Verification items for the finished model (mm, model axes). A direction names the side the tool comes from. Give positions to 0.01 mm unless a question says otherwise; leave off trailing zeros. Order: outer loops, then holes, each group sorted by start corner. A loop starts at its lowest first (then second) coordinate and runs counter-clockwise, first axis right, second up. Notation, with made-up numbers: (31, -29.75) -> (63, -29.75) arc R13 cw to (63, -24.75) -> close; hole circle Ø8 at (72, 3). An arc over 180 degrees is marked (long way). One line per question, with ' | ' between items. Start each with the question number.
Q1. Section check B-B on x = -33. Record the cut outline in (y, z), plus the area to 3 significant figures.
Q2. Section check D-D on z = -13. Record the cut outline in (x, y).
Q3. Go/stop test with flat-tipped pins: pin 1 (0.6 mm diameter, centred on y = -26, z = -15, fed in from +X); pin 2 (4 mm diameter, centred on x = -44.5, y = -23, fed in from +Z); pin 3 (0.9 mm diameter, centred on y = -26.5, z = -17, fed in from -X). Record where each tip stops, or that it passes through.
Q4. Material ranges on probe 1 along X at (y, z) = (-9, -14.5); probe 2 along Y at (x, z) = (-40, -10.25); probe 3 along Y at (x, z) = (9, -19.5), recorded low to high. Write a range as [from, to].
Q5. Section check C-C on z = -7.75. Record the cut outline in (x, y), plus the area to 3 significant figures.
Q6. Section check A-A on y = 3.5. Record the cut outline in (x, z), plus the area to 3 significant figures.
Q7. Mould release check, pull along Y, two halves, no side actions. Record for faces 1 (the flat face through (-44, -21, -11.25)), 2 (the flat face through (-49, 1, -2)), 3 (the flat face through (-44, 22.7, -11.25)), 4 (the flat face through (-10, 28.924, -11)): released by +Y, released by -Y, zero draft, split by the parting line, or undercut.
Q8. Access from +Z, -Z, +X, -X, +Y, -Y to the whole of each face (thin tool, end or side, straight path). Record for faces 5 (the flat face through (-10, -25.976, -20)), 6 (the flat face through (29.665, 0, -3)), 7 (the cylindrical face through (-43.843, 24.1, -15.071)), 8 (the flat face through (31.165, 0, -11)), 9 (the flat face through (-7, -26, -18.312)).
from build123d import *

# Parameters (mm, degrees)
BOSS_EXTRUDE1_START = -2
SKETCH1_W           = 81.4
SKETCH1_H           = 56.4
SKETCH1_W_2         = 75.4
SKETCH1_H_2         = 50.4
BOSS_EXTRUDE1_DEPTH = 27
FILLET1_R           = 3
SKETCH2_R           = 1.3
CUT_EXTRUDE1_DEPTH  = 2
CUT_EXTRUDE2_START  = -17
SKETCH2_3_R         = 1.3
CUT_EXTRUDE2_DEPTH  = 10
BOSS_EXTRUDE2_START = -7.25
SKETCH3_R           = 1.25
BOSS_EXTRUDE2_DEPTH = 7.75
CUT_EXTRUDE3_DEPTH  = 28.2
CUT_EXTRUDE4_START  = -8
CUT_EXTRUDE4_DEPTH  = 8


with BuildPart() as part:
    # Sketch1 → Boss-Extrude1 (new body)
    with BuildSketch(Plane.XY.offset(BOSS_EXTRUDE1_START)):
        with Locations((-9.535141298, 0.724362859)):
            Rectangle(SKETCH1_W, SKETCH1_H)
        with Locations((-9.535141298, 0.724362859)):
            Rectangle(SKETCH1_W_2, SKETCH1_H_2, mode=Mode.SUBTRACT)
    extrude(amount=-BOSS_EXTRUDE1_DEPTH)

    # Fillet1
    fillet1_edges = [part.edges().sort_by_distance(p)[0] for p in [
        (-50.235141298, -27.475637141, -15.5),
        (-50.235141298, 28.924362859, -15.5),
        (31.164858702, 28.924362859, -15.5),
        (31.164858702, -27.475637141, -15.5),
    ]]
    fillet(fillet1_edges, radius=FILLET1_R)

    # Sketch2 → Cut-Extrude1 (cut)
    with BuildSketch(Plane.XY.offset(-2)):
        with Locations((25.964858702, -22.275637141)):
            Circle(SKETCH2_R)
        with BuildLine():
            Line((28.164858702, 27.424362859), (-47.235141298, 27.424362859))
            ThreePointArc((-47.235141298, 27.424362859), (-48.29580147, 26.985023031), (-48.735141298, 25.924362859))
            Line((-48.735141298, 25.924362859), (-48.735141298, -24.475637141))
            ThreePointArc((-48.735141298, -24.475637141), (-48.29580147, -25.536297313), (-47.235141298, -25.975637141))
            Line((-47.235141298, -25.975637141), (28.164858702, -25.975637141))
            ThreePointArc((28.164858702, -25.975637141), (29.225518873, -25.536297313), (29.664858702, -24.475637141))
            Line((29.664858702, -24.475637141), (29.664858702, 25.924362859))
            ThreePointArc((29.664858702, 25.924362859), (29.225518873, 26.985023031), (28.164858702, 27.424362859))
        make_face()
    extrude(amount=-CUT_EXTRUDE1_DEPTH, mode=Mode.SUBTRACT)

    # Sketch2<3> → Cut-Extrude2 (cut)
    with BuildSketch(Plane.XY.offset(-2).offset(CUT_EXTRUDE2_START)):
        with BuildLine():
            Line((28.164858702, 27.424362859), (-47.235141298, 27.424362859))
            ThreePointArc((-47.235141298, 27.424362859), (-48.29580147, 26.985023031), (-48.735141298, 25.924362859))
            Line((-48.735141298, 25.924362859), (-48.735141298, -24.475637141))
            ThreePointArc((-48.735141298, -24.475637141), (-48.29580147, -25.536297313), (-47.235141298, -25.975637141))
            Line((-47.235141298, -25.975637141), (28.164858702, -25.975637141))
            ThreePointArc((28.164858702, -25.975637141), (29.225518873, -25.536297313), (29.664858702, -24.475637141))
            Line((29.664858702, -24.475637141), (29.664858702, 25.924362859))
            ThreePointArc((29.664858702, 25.924362859), (29.225518873, 26.985023031), (28.164858702, 27.424362859))
        make_face()
        with Locations((25.964858702, 23.724362859)):
            Circle(SKETCH2_3_R, mode=Mode.SUBTRACT)
        with Locations((-45.035141298, 23.724362859)):
            Circle(SKETCH2_3_R, mode=Mode.SUBTRACT)
        with Locations((-45.035141298, -22.275637141)):
            Circle(SKETCH2_3_R, mode=Mode.SUBTRACT)
        with Locations((25.964858702, -22.275637141)):
            Circle(SKETCH2_3_R, mode=Mode.SUBTRACT)
    extrude(amount=-CUT_EXTRUDE2_DEPTH, mode=Mode.SUBTRACT)

    # Sketch3 → Boss-Extrude2 (add)
    # profile 1 of 4: a face of its own
    with BuildSketch(Plane.XY.offset(-4).offset(BOSS_EXTRUDE2_START)):
        with BuildLine():
            Line((-47.235141298, -24.475637141), (-42.835141298, -24.475637141))
            ThreePointArc((-42.835141298, -24.475637141), (-42.160702776, -23.466268561), (-41.923871461, -22.275637141))
            ThreePointArc((-41.923871461, -22.275637141), (-43.844509878, -19.401198618), (-47.235141298, -20.075637141))
            Line((-47.235141298, -20.075637141), (-47.235141298, -24.475637141))
        make_face()
        with Locations((-45.035141298, -22.275637141)):
            Circle(SKETCH3_R, mode=Mode.SUBTRACT)
    # profile 2 of 4: a face of its own
    with BuildSketch(Plane.XY.offset(-4).offset(BOSS_EXTRUDE2_START)):
        with BuildLine():
            ThreePointArc((-41.923871461, 23.724362859), (-42.160702776, 24.914994279), (-42.835141298, 25.924362859))
            Line((-42.835141298, 25.924362859), (-47.235141298, 25.924362859))
            Line((-47.235141298, 25.924362859), (-47.235141298, 21.524362859))
            ThreePointArc((-47.235141298, 21.524362859), (-43.844509878, 20.849924336), (-41.923871461, 23.724362859))
        make_face()
        with Locations((-45.035141298, 23.724362859)):
            Circle(SKETCH3_R, mode=Mode.SUBTRACT)
    # profile 3 of 4: a face of its own
    with BuildSketch(Plane.XY.offset(-4).offset(BOSS_EXTRUDE2_START)):
        with BuildLine():
            ThreePointArc((23.764858702, 25.924362859), (23.764858702, 21.524362859), (28.164858702, 21.524362859))
            Line((28.164858702, 21.524362859), (28.164858702, 25.924362859))
            Line((28.164858702, 25.924362859), (23.764858702, 25.924362859))
        make_face()
        with Locations((25.964858702, 23.724362859)):
            Circle(SKETCH3_R, mode=Mode.SUBTRACT)
    # profile 4 of 4: a face of its own
    with BuildSketch(Plane.XY.offset(-4).offset(BOSS_EXTRUDE2_START)):
        with BuildLine():
            Line((23.764858702, -24.475637141), (28.164858702, -24.475637141))
            Line((28.164858702, -24.475637141), (28.164858702, -20.075637141))
            ThreePointArc((28.164858702, -20.075637141), (23.764858702, -20.075637141), (23.764858702, -24.475637141))
        make_face()
        with Locations((25.964858702, -22.275637141)):
            Circle(SKETCH3_R, mode=Mode.SUBTRACT)
    extrude(amount=-BOSS_EXTRUDE2_DEPTH)

    # Sketch5 → Cut-Extrude3 (cut)
    with BuildSketch(Plane.XZ.offset(27.475637141)):
        with BuildLine():
            Line((-10.285143265, -18.312481798), (-3.785143265, -18.312481798))
            ThreePointArc((-3.785143265, -18.312481798), (-3.184102501, -18.063522562), (-2.935143265, -17.462481798))
            Line((-2.935143265, -17.462481798), (-2.935143265, -16.642481798))
            ThreePointArc((-2.935143265, -16.642481798), (-3.025595699, -16.260922505), (-3.277702075, -15.960570192))
            Line((-3.277702075, -15.960570192), (-3.489691711, -15.80281914))
            ThreePointArc((-3.489691711, -15.80281914), (-3.534181071, -15.749815791), (-3.550143265, -15.682481798))
            Line((-3.550143265, -15.682481798), (-3.550143265, -14.962481798))
            ThreePointArc((-3.550143265, -14.962481798), (-3.799102501, -14.361441034), (-4.400143265, -14.112481798))
            Line((-4.400143265, -14.112481798), (-9.670143265, -14.112481798))
            ThreePointArc((-9.670143265, -14.112481798), (-10.271184029, -14.361441034), (-10.520143265, -14.962481798))
            Line((-10.520143265, -14.962481798), (-10.520143265, -15.682481798))
            ThreePointArc((-10.520143265, -15.682481798), (-10.53610546, -15.749815791), (-10.58059482, -15.80281914))
            Line((-10.58059482, -15.80281914), (-10.792584456, -15.960570192))
            ThreePointArc((-10.792584456, -15.960570192), (-11.044690832, -16.260922505), (-11.135143265, -16.642481798))
            Line((-11.135143265, -16.642481798), (-11.135143265, -17.462481798))
            ThreePointArc((-11.135143265, -17.462481798), (-10.886184029, -18.063522562), (-10.285143265, -18.312481798))
        make_face()
    extrude(amount=-CUT_EXTRUDE3_DEPTH, mode=Mode.SUBTRACT)

    # Sketch6 → Cut-Extrude4 (cut)
    with BuildSketch(Plane(origin=(0, 0, -29), x_dir=(-1, 0, 0), z_dir=(0, 0, -1)).offset(CUT_EXTRUDE4_START)):
        with BuildLine():
            Line((50.235141298, -24.475637141), (50.235141298, 25.924362859))
            ThreePointArc((50.235141298, 25.924362859), (49.356461642, 28.045683202), (47.235141298, 28.924362859))
            Line((47.235141298, 28.924362859), (-28.164858702, 28.924362859))
            ThreePointArc((-28.164858702, 28.924362859), (-30.286179045, 28.045683202), (-31.164858702, 25.924362859))
            Line((-31.164858702, 25.924362859), (-31.164858702, -24.475637141))
            ThreePointArc((-31.164858702, -24.475637141), (-30.286179045, -26.596957485), (-28.164858702, -27.475637141))
            Line((-28.164858702, -27.475637141), (47.235141298, -27.475637141))
            ThreePointArc((47.235141298, -27.475637141), (49.356461642, -26.596957485), (50.235141298, -24.475637141))
        make_face()
        with BuildLine():
            Line((-29.664858702, 25.924362859), (-29.664858702, -24.475637141))
            ThreePointArc((-29.664858702, -24.475637141), (-29.225518873, -25.536297313), (-28.164858702, -25.975637141))
            Line((-28.164858702, -25.975637141), (47.235141298, -25.975637141))
            ThreePointArc((47.235141298, -25.975637141), (48.29580147, -25.536297313), (48.735141298, -24.475637141))
            Line((48.735141298, -24.475637141), (48.735141298, 25.924362859))
            ThreePointArc((48.735141298, 25.924362859), (48.29580147, 26.985023031), (47.235141298, 27.424362859))
            Line((47.235141298, 27.424362859), (-28.164858702, 27.424362859))
            ThreePointArc((-28.164858702, 27.424362859), (-29.225518873, 26.985023031), (-29.664858702, 25.924362859))
        make_face(mode=Mode.SUBTRACT)
    extrude(amount=CUT_EXTRUDE4_DEPTH, mode=Mode.SUBTRACT)


solid = part.part
Filled in:
1) outline: (-27.48, -21) -> (-25.98, -21) -> (-25.98, -19) -> (-24.48, -19) -> (-24.48, -4) -> (-25.98, -4) -> (-25.98, -2) -> (-27.48, -2) -> close; (25.92, -19) -> (27.42, -19) -> (27.42, -21) -> (28.92, -21) -> (28.92, -2) -> (27.42, -2) -> (27.42, -4) -> (25.92, -4) -> close | area: 102 mm²
2) outline: (-50.24, -24.48) arc R3 ccw to (-47.24, -27.48) -> (28.16, -27.48) arc R3 ccw to (31.16, -24.48) -> (31.16, 25.92) arc R3 ccw to (28.16, 28.92) -> (-47.24, 28.92) arc R3 ccw to (-50.24, 25.92) -> close; hole (-47.24, -20.08) arc R3.11 cw to (-42.84, -24.48) -> (23.76, -24.48) arc R3.11 cw to (28.16, -20.08) -> (28.16, 21.52) arc R3.11 cw to (23.76, 25.92) -> (-42.84, 25.92) arc R3.11 cw to (-47.24, 21.52) -> close; hole circle Ø2.5 at (-45.04, -22.28); hole circle Ø2.5 at (-45.04, 23.72); hole circle Ø2.5 at (25.96, -22.28); hole circle Ø2.5 at (25.96, 23.72)
3) pin 1: x = 30.9 | pin 2: z = -4 | pin 3: x = -49.79
4) probe 1: [-50.24, -47.24], [28.16, 31.16] | probe 2: [-27.48, -24.48], [25.92, 28.92] | probe 3: [-27.48, -25.98], [27.42, 28.92]
5) outline: (-50.24, -24.48) arc R3 ccw to (-47.24, -27.48) -> (28.16, -27.48) arc R3 ccw to (31.16, -24.48) -> (31.16, 25.92) arc R3 ccw to (28.16, 28.92) -> (-47.24, 28.92) arc R3 ccw to (-50.24, 25.92) -> close; hole (-47.24, -24.48) -> (28.16, -24.48) -> (28.16, 25.92) -> (-47.24, 25.92) -> close | area: 783 mm²
6) outline: (-50.24, -21) -> (-48.74, -21) -> (-48.74, -19) -> (-47.24, -19) -> (-47.24, -4) -> (-48.74, -4) -> (-48.74, -2) -> (-50.24, -2) -> close; (28.16, -19) -> (29.66, -19) -> (29.66, -21) -> (31.16, -21) -> (31.16, -2) -> (29.66, -2) -> (29.66, -4) -> (28.16, -4) -> close | area: 102 mm²
7) face 1: undercut | face 2: zero draft | face 3: undercut | face 4: released by +Y
8) face 5: -Z | face 6: +Z | face 7: +Z, -Z | face 8: +Z, -Z, +X, +Y, -Y | face 9: -Y
